Part print with two shaded views. Sizes in mm from the minimum x, y, z corner. A direction names the side the tool comes from. Round coordinates to 2 decimals unless told otherwise and drop trailing zeros. Order: outer loops, then holes, each group sorted by start corner. A loop starts at its lowest first (then second) coordinate and runs counter-clockwise, first axis right, second up. Notation, with made-up numbers: (4.25, 26.25) -> (51.25, 26.25) arc R21 cw to (51.25, 30.25) -> close; hole circle Ø10 at (12.5, 75.5). An arc over 180 degrees is marked (long way). Put each result on its own line as item: value. Start each with the question number.
Q1. Cut at A-A, the plane x = 20. List the corners of the cut face in (y, z).
Q2. Flat gauge pins, fed straight in: P1, Ø4, axis at x = 20, y = 2.5, coming from the -Z side; P2, Ø2, axis at y = 5.5, z = 7, coming from the -X side (1 decimal); P3, Ø1.5, axis at x = 16, z = 4, coming from the +Y side. Where does each tip first touch, or does it go through?
Q3. Probe L1, parallel to X at y = 11.25, z = 6.75 (1 decimal); L2, parallel to Z at x = 8, y = 5; L3, parallel to X at y = 21, z = 6.25 (1 decimal). List the from-to ranges inside material, lowest first.
Q4. Cut at C-C, the plane y = 28.75. List the corners of the cut face in (x, z) (1 decimal).
Q5. Pull direction X, two halves, no side cores. Call the marked faces 4, 5 and 6: released by +X, released by -X, zero draft, split by the parting line, or undercut.
Q6. 3-axis set-ups, long thin cutter, end or side, ignore diameter. For the marked faces 1, 2 and 3: which of +Z, -Z, +X, -X, +Y, -Y reach the whole face in a straight line?
Q7. Cut at B-B, the plane y = 20. List the corners of the cut face in (x, z), and give its area (3 significant figures).
Q8. Cut at D-D, the plane z = 2. List the corners of the cut face in (x, y).
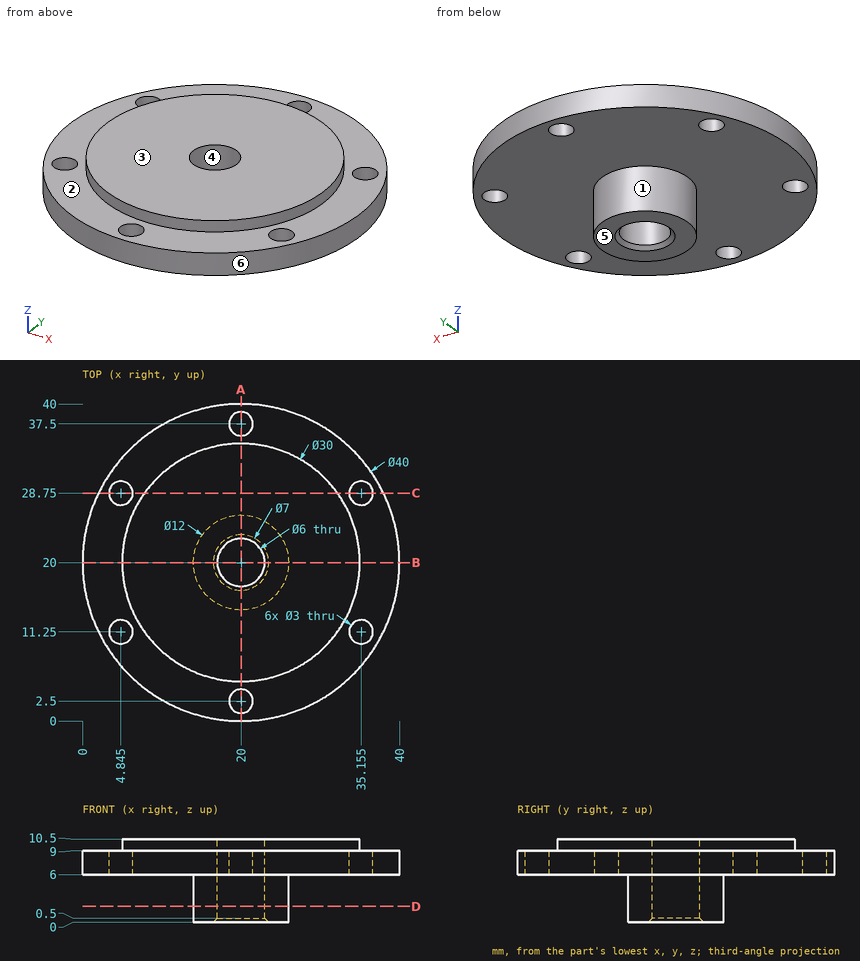
Ans:
1. outline: (0, 6) -> (1, 6) -> (1, 9) -> (0, 9) -> close; (4, 6) -> (14, 6) -> (14, 0) -> (16.5, 0) -> (17, 0.5) -> (17, 10.5) -> (5, 10.5) -> (5, 9) -> (4, 9) -> close; (23, 0.5) -> (23.5, 0) -> (26, 0) -> (26, 6) -> (36, 6) -> (36, 9) -> (35, 9) -> (35, 10.5) -> (23, 10.5) -> close; (39, 6) -> (40, 6) -> (40, 9) -> (39, 9) -> close
2. P1: stops at z = 6
2. P2: stops at x = 5.2
2. P3: stops at y = 25.04
3. L1: x = 2 to 3.3, 6.3 to 33.7, 36.7 to 38
3. L2: z = 6 to 9
3. L3: x = 0 to 17.2, 22.8 to 40
4. outline: (2, 6) -> (3.3, 6) -> (3.3, 9) -> (2, 9) -> close; (6.3, 6) -> (33.7, 6) -> (33.7, 9) -> (32.2, 9) -> (32.2, 10.5) -> (7.8, 10.5) -> (7.8, 9) -> (6.3, 9) -> close; (36.7, 6) -> (38, 6) -> (38, 9) -> (36.7, 9) -> close
5. face 4: undercut
5. face 5: zero draft
5. face 6: split by the parting line
6. face 1: -Z
6. face 2: +Z
6. face 3: +Z, +X, -X, +Y, -Y
7. outline: (0, 6) -> (14, 6) -> (14, 0) -> (16.5, 0) -> (17, 0.5) -> (17, 10.5) -> (5, 10.5) -> (5, 9) -> (0, 9) -> close; (23, 0.5) -> (23.5, 0) -> (26, 0) -> (26, 6) -> (40, 6) -> (40, 9) -> (35, 9) -> (35, 10.5) -> (23, 10.5) -> close
7. area: 174 mm^2
8. outline: circle Ø12 at (20, 20); hole circle Ø6 at (20, 20)
